```python
from build123d import *

# Parameters (mm, degrees)
SKIZZE1_W                       = 230
SKIZZE1_H                       = 90
AUFSATZ_LINEAR_AUSTRAGEN1_DEPTH = 15
F_7_0_7_DURCHMESSER_BOHRUNG1_D  = 7
VERRUNDUNG3_R                   = 2
VERRUNDUNG4_R                   = 2


with BuildPart() as part:
    # Skizze1 → Aufsatz-Linear austragen1 (new body)
    with BuildSketch(Plane.XY):
        Rectangle(SKIZZE1_W, SKIZZE1_H)
    extrude(amount=AUFSATZ_LINEAR_AUSTRAGEN1_DEPTH)

    # Ø7.0 (7) Durchmesser Bohrung1 (through all)
    with Locations(Plane.XY.offset(15)):
        with Locations((100, -30), (-100, -30), (-100, 30), (100, 30)):
            Hole(F_7_0_7_DURCHMESSER_BOHRUNG1_D / 2)

    # Verrundung3
    verrundung3_edges = [part.edges().sort_by_distance(p)[0] for p in [
        (-115, 45, 7.5),
        (115, 45, 7.5),
    ]]
    fillet(verrundung3_edges, radius=VERRUNDUNG3_R)

    # Verrundung4
    verrundung4_edges = [part.edges().sort_by_distance(p)[0] for p in [
        (115, -45, 7.5),
        (-115, -45, 7.5),
    ]]
    fillet(verrundung4_edges, radius=VERRUNDUNG4_R)


solid = part.part
```
The model under review builds one solid part; all positions refer to its coordinate system, in mm. Round coordinates to 2 decimals unless told otherwise and drop trailing zeros. Loops run counter-clockwise (first coordinate to the right, second up) from the corner with the lowest first, then second, coordinate; pieces in that order, holes last.
1) Wall thickness on line 1 along Y through (x, z) = (100, 4.5); line 2 along X through (y, z) = (-28.5, 1.75): over which ranges is each line inside the solid? List them lowest first.
Values follow:
line 1: y = -45 to -33.5, -26.5 to 26.5, 33.5 to 45
line 2: x = -115 to -103.16, -96.84 to 96.84, 103.16 to 115
2) Clearance check with a flat-ended pin moving along its axis: P1, Ø4, axis at x = -100, y = 30, coming from the -Z side. State where the tip first meets the part, or that it passes through.
Values follow:
P1: passes through
3) The part is to be moulded in two halves that separate along Y. For faces 1 (the face through (-2, 1, 15)), 2 (the face through (-2, 45, 7)), 3 (the face through (-103.34, -28.95, 7.4)), say which applies: pulls with the +Y half, pulls with the -Y half, needs draft (parallel to the pull), parting line crosses it, or undercut.
Values follow:
face 1: needs draft
face 2: pulls with the +Y half
face 3: undercut
4) Consider section B-B on y = -30. State the section outline as (x, z) points, then the cut area to 3 significant figures.
Values follow:
outline: (-115, 0) - (-103.5, 0) - (-103.5, 15) - (-115, 15) - close; (-96.5, 0) - (96.5, 0) - (96.5, 15) - (-96.5, 15) - close; (103.5, 0) - (115, 0) - (115, 15) - (103.5, 15) - close
area: 3,240 mm2
5) Consider section A-A on x = -100. State the section outline as (y, z) points, then the cut area to 3 significant figures.
Values follow:
outline: (-45, 0) - (-33.5, 0) - (-33.5, 15) - (-45, 15) - close; (-26.5, 0) - (26.5, 0) - (26.5, 15) - (-26.5, 15) - close; (33.5, 0) - (45, 0) - (45, 15) - (33.5, 15) - close
area: 1,140 mm2
